Can you work these out from the model? Positions are in its coordinate system, mm. A direction names the side the tool comes from. Round coordinates to 2 decimals unless told otherwise and drop trailing zeros. Loops run counter-clockwise (first coordinate to the right, second up) from the corner with the lowest first, then second, coordinate; pieces in that order, holes last.
from build123d import *

# Parameters (mm, degrees)
F1_DEPTH = 25.4
F2_T     = -3.175
F3_DEPTH = 25.4
F5_DEPTH = 3.175
F6_R     = 3.175
F7_DEPTH = 25.4
F9_DEPTH = 3.175


# Not quite as in the source:
# - a feature names something its author has since deleted; it is built from what else it names


with BuildPart() as f1:
    # F0 (on Top) → F1 (new body)
    with BuildSketch(Plane.XY):
        Polygon((11.90625, 11.90625), (-11.90625, 11.90625), (-11.90625, -11.90625), align=None)
    extrude(amount=F1_DEPTH)

    # F2
    f2_openings = [f1.faces().sort_by_distance(p)[0] for p in [
        (-11.90625, 0, 12.7),
    ]]
    offset(amount=F2_T, openings=f2_openings)

    # F3 (cut): a face of the model
    f3_faces = [f1.faces().sort_by_distance(p)[0] for p in [
        (-6.5237926868, 3.3487926868, 3.175),
    ]]
    extrude(f3_faces, amount=-F3_DEPTH, mode=Mode.SUBTRACT)

    # F4 (on face) → F5 (cut)
    with BuildSketch(Plane(origin=(-11.90625, 0, 0), x_dir=(0, -1, 0), z_dir=(-1, 0, 0))):
        with BuildLine():
            ThreePointArc((3.175, 12.7), (2.9133467904, 13.962155093), (2.1715130842, 15.0162806231))
            Line((2.1715130842, 15.0162806231), (0, 12.7))
            Line((0, 12.7), (2.1715130842, 10.3837193769))
            ThreePointArc((2.1715130842, 10.3837193769), (2.9133467904, 11.437844907), (3.175, 12.7))
        make_face()
        with BuildLine():
            Line((0, 12.7), (2.1715130842, 15.0162806231))
            ThreePointArc((2.1715130842, 15.0162806231), (0, 15.875), (-2.1715130842, 15.0162806231))
            Line((-2.1715130842, 15.0162806231), (0, 12.7))
        make_face()
        with BuildLine():
            Line((-2.1715130842, 10.3837193769), (0, 12.7))
            Line((0, 12.7), (-2.1715130842, 15.0162806231))
            ThreePointArc((-2.1715130842, 15.0162806231), (-3.175, 12.7), (-2.1715130842, 10.3837193769))
        make_face()
        with BuildLine():
            Line((2.1715130842, 10.3837193769), (0, 12.7))
            Line((0, 12.7), (-2.1715130842, 10.3837193769))
            ThreePointArc((-2.1715130842, 10.3837193769), (0, 9.525), (2.1715130842, 10.3837193769))
        make_face()
    extrude(amount=-F5_DEPTH, mode=Mode.SUBTRACT)

    # F6 (on face) → F7 (cut)
    with BuildSketch(Plane.XY.offset(25.4)):
        with Locations((-7.46125, 2.38125)):
            Circle(F6_R)
    extrude(amount=-F7_DEPTH, mode=Mode.SUBTRACT)

    # F8 (on face) → F9 (cut)
    with BuildSketch(Plane(origin=(0, 0, 0), x_dir=(0.7071067812, 0.7071067812, 0), z_dir=(0.7071067812, -0.7071067812, 0))):
        with BuildLine():
            ThreePointArc((3.175, 12.7), (1.0081076412, 15.7107048982), (-2.5348229819, 14.6118832209))
            Line((-2.5348229819, 14.6118832209), (2.5348229819, 10.7881167791))
            ThreePointArc((2.5348229819, 10.7881167791), (3.0107048982, 11.6918923588), (3.175, 12.7))
        make_face()
        with BuildLine():
            Line((2.5348229819, 10.7881167791), (-2.5348229819, 14.6118832209))
            ThreePointArc((-2.5348229819, 14.6118832209), (-1.9118832209, 10.1651770181), (2.5348229819, 10.7881167791))
        make_face()
    extrude(amount=-F9_DEPTH, mode=Mode.SUBTRACT)


solid = f1.part
(1) If we section it at B-B, the plane z = 4.25: List the corners of the cut face in (x, y) for me.
Worked answers:
outline: (-11.91, -11.91) - (11.91, 11.91) - (-11.91, 11.91) - (-11.91, 8.73) - (4.24, 8.73) - (-11.91, -7.42) - close
(2) If we section it at A-A, the plane x = -5.5: List the corners of the cut face in (y, z) for me (3 decimals), then the cut area to 3 significant figures.
Worked answers:
outline: (-5.5, 0) - (-1.01, 0) - (-1.01, 22.225) - (-0.116, 22.225) - (-0.116, 25.4) - (-5.5, 25.4) - close; (4.878, 22.225) - (8.731, 22.225) - (8.731, 0) - (11.906, 0) - (11.906, 25.4) - (4.878, 25.4) - close
area: 210 mm2
(3) For faces 4 (the flat face through (-3.95, 0.54, 8.49)), 5 (the flat face through (2.5, 2.5, 12.5)), which set-ups out of +Z, -Z, +X, -X, +Y, -Y let a thin tool reach every point of the face, with its end or its side?
Worked answers:
face 4: -Z, -X
face 5: +Z, -Z, +X, -Y
(4) Will these pins go through, and if not, where does the flat tip stop? P1, Ø2, axis at y = 2.5, z = 13, coming from the -X side; P2, Ø4, axis at x = -4.5, z = 14.5, coming from the -Y side; P3, Ø13, axis at x = -7.5, z = 8, coming from the -Y side.
Worked answers:
P1: stops at x = 0.95
P2: stops at y = -6.5
P3: stops at y = -11.91
(5) If we section it at C-C, the plane x = 3: List the corners of the cut face in (y, z) for me (3 decimals).
Worked answers:
outline: (3, 0) - (7.49, 0) - (7.49, 22.225) - (8.731, 22.225) - (8.731, 0) - (11.906, 0) - (11.906, 25.4) - (3, 25.4) - close
(6) If I drill on line 1 (Y direction, x = 0, z = 19.5); line 2 (Y direction, x = -3.75, z = 3); line 3 (Y direction, x = 8.25, z = 18.5), over which ranges is the centre line in solid material (lowest first)?
Worked answers:
line 1: y = 0 to 4.49, 8.73 to 11.91
line 2: y = -3.75 to 0.74, 8.73 to 11.91
line 3: y = 8.25 to 11.91
(7) If we mould it in two halves opening along Y, with no side actions, what happens to faces 1 (the flat face through (0, 11.906, 13)), 2 (the flat face through (-4, 8.731, 11)), 3 (the flat face through (-11.906, -8, 15))? For each: released by +Y, released by -Y, zero draft, split by the parting line, or undercut.
Worked answers:
face 1: released by +Y
face 2: undercut
face 3: zero draft
(8) If we section it at D-D, the plane y = 9.25: List the corners of the cut face in (x, z) for me.
Worked answers:
outline: (-11.91, 0) - (9.25, 0) - (9.25, 25.4) - (-11.91, 25.4) - close
